```python
from build123d import *

# Parameters (mm, degrees)
SKETCH1_R           = 1.5
BOSS_EXTRUDE1_DEPTH = 5
SKETCH2_R           = 2
CUT_EXTRUDE1_DEPTH  = 5
FILLET1_R           = 7
FILLET2_R           = 7
FILLET3_R           = 3


with BuildPart() as part:
    # Sketch1 → Boss-Extrude1 (new body)
    with BuildSketch(Plane.XY):
        Polygon((33, 0), (195.6, 0), (195.6, -70), (228.6, -70), (228.6, -158.6), (195.6, -158.6), (195.6, -228.6), (33, -228.6), (33, -158.6), (0, -158.6), (0, -70), (33, -70), align=None)
        with Locations((95.3, -32)):
            Circle(SKETCH1_R, mode=Mode.SUBTRACT)
        with Locations((133.3, -32)):
            Circle(SKETCH1_R, mode=Mode.SUBTRACT)
        with Locations((39, -21.625)):
            Circle(SKETCH1_R, mode=Mode.SUBTRACT)
        with Locations((39, -38.375)):
            Circle(SKETCH1_R, mode=Mode.SUBTRACT)
        with Locations((54, -38.375)):
            Circle(SKETCH1_R, mode=Mode.SUBTRACT)
        with Locations((54, -21.625)):
            Circle(SKETCH1_R, mode=Mode.SUBTRACT)
        with Locations(Location((54, -206.975, 0), (0, 0, 180))):
            Circle(SKETCH1_R, mode=Mode.SUBTRACT)
        with Locations(Location((54, -190.225, 0), (0, 0, 180))):
            Circle(SKETCH1_R, mode=Mode.SUBTRACT)
        with Locations(Location((39, -190.225, 0), (0, 0, 180))):
            Circle(SKETCH1_R, mode=Mode.SUBTRACT)
        with Locations(Location((39, -206.975, 0), (0, 0, 180))):
            Circle(SKETCH1_R, mode=Mode.SUBTRACT)
        with Locations((174.6, -190.225)):
            Circle(SKETCH1_R, mode=Mode.SUBTRACT)
        with Locations((174.6, -206.975)):
            Circle(SKETCH1_R, mode=Mode.SUBTRACT)
        with Locations((189.6, -206.975)):
            Circle(SKETCH1_R, mode=Mode.SUBTRACT)
        with Locations((189.6, -190.225)):
            Circle(SKETCH1_R, mode=Mode.SUBTRACT)
        with Locations(Location((189.6, -38.375, 0), (0, 0, 180))):
            Circle(SKETCH1_R, mode=Mode.SUBTRACT)
        with Locations(Location((174.6, -38.375, 0), (0, 0, 180))):
            Circle(SKETCH1_R, mode=Mode.SUBTRACT)
        with Locations(Location((174.6, -21.625, 0), (0, 0, 180))):
            Circle(SKETCH1_R, mode=Mode.SUBTRACT)
        with Locations(Location((189.6, -21.625, 0), (0, 0, 180))):
            Circle(SKETCH1_R, mode=Mode.SUBTRACT)
        with BuildLine():
            Line((72.264776933, -37.198562168), (72.264776933, -22.801437832))
            ThreePointArc((72.264776933, -22.801437832), (77.438501315, -17.627713451), (82.612225696, -22.801437832))
            Line((82.612225696, -22.801437832), (82.612225696, -37.198562168))
            ThreePointArc((82.612225696, -37.198562168), (77.438501315, -42.372286549), (72.264776933, -37.198562168))
        make_face(mode=Mode.SUBTRACT)
        with BuildLine():
            Line((103.657302093, -26.446561828), (124.942697907, -26.446561828))
            ThreePointArc((124.942697907, -26.446561828), (130.496136079, -32), (124.942697907, -37.553438172))
            Line((124.942697907, -37.553438172), (103.657302093, -37.553438172))
            ThreePointArc((103.657302093, -37.553438172), (98.103863921, -32), (103.657302093, -26.446561828))
        make_face(mode=Mode.SUBTRACT)
        with BuildLine():
            Line((72.264776933, -191.401437832), (72.264776933, -205.798562168))
            ThreePointArc((72.264776933, -205.798562168), (77.438501315, -210.972286549), (82.612225696, -205.798562168))
            Line((82.612225696, -205.798562168), (82.612225696, -191.401437832))
            ThreePointArc((82.612225696, -191.401437832), (77.438501315, -186.227713451), (72.264776933, -191.401437832))
        make_face(mode=Mode.SUBTRACT)
        with BuildLine():
            Line((156.335223067, -191.401437832), (156.335223067, -205.798562168))
            ThreePointArc((156.335223067, -205.798562168), (151.161498685, -210.972286549), (145.987774304, -205.798562168))
            Line((145.987774304, -205.798562168), (145.987774304, -191.401437832))
            ThreePointArc((145.987774304, -191.401437832), (151.161498685, -186.227713451), (156.335223067, -191.401437832))
        make_face(mode=Mode.SUBTRACT)
        with BuildLine():
            Line((156.335223067, -37.198562168), (156.335223067, -22.801437832))
            ThreePointArc((156.335223067, -22.801437832), (151.161498685, -17.627713451), (145.987774304, -22.801437832))
            Line((145.987774304, -22.801437832), (145.987774304, -37.198562168))
            ThreePointArc((145.987774304, -37.198562168), (151.161498685, -42.372286549), (156.335223067, -37.198562168))
        make_face(mode=Mode.SUBTRACT)
    extrude(amount=BOSS_EXTRUDE1_DEPTH)

    # Sketch2 → Cut-Extrude1 (cut)
    with BuildSketch(Plane.XY.offset(5)):
        with Locations((54.3, -59.307305139)):
            Circle(SKETCH2_R)
        with Locations(Location((174.3, -59.307305139, 0), (0, 0, 180))):
            Circle(SKETCH2_R)
        with Locations((174.3, -169.292694861)):
            Circle(SKETCH2_R)
        with Locations(Location((54.3, -169.292694861, 0), (0, 0, 180))):
            Circle(SKETCH2_R)
    extrude(amount=-CUT_EXTRUDE1_DEPTH, mode=Mode.SUBTRACT)

    # Fillet1
    fillet1_edges = [part.edges().sort_by_distance(p)[0] for p in [
        (33, 0, 2.5),
        (195.6, 0, 2.5),
        (228.6, -70, 2.5),
        (228.6, -158.6, 2.5),
        (0, -158.6, 2.5),
        (0, -70, 2.5),
    ]]
    fillet(fillet1_edges, radius=FILLET1_R)

    # Fillet2
    fillet2_edges = [part.edges().sort_by_distance(p)[0] for p in [
        (195.6, -228.6, 2.5),
        (33, -228.6, 2.5),
    ]]
    fillet(fillet2_edges, radius=FILLET2_R)

    # Fillet3
    fillet3_edges = [part.edges().sort_by_distance(p)[0] for p in [
        (33, -70, 2.5),
        (195.6, -70, 2.5),
        (195.6, -158.6, 2.5),
        (33, -158.6, 2.5),
    ]]
    fillet(fillet3_edges, radius=FILLET3_R)


solid = part.part
```
Geometry check sheet. Reference: the model listing, model coordinates, mm. A direction names the side the tool comes from. Coordinates: 2 decimals unless noted, no trailing zeros. Order: outer loops, then holes, each group sorted by start corner. A loop starts at its lowest first (then second) coordinate and runs counter-clockwise, first axis right, second up. Notation, with made-up numbers: (59, 43.5) - (116, 43.5) arc R18 cw to (116, 53.5) - close; hole circle Ø1 at (-6.5, 33). An arc over 180 degrees is marked (long way). Answer in a Markdown table with one row per item. Add a question column.
1. Section check C-C (x = 26.5). Enter the section's corners in (y, z).
2. Access from +Z, -Z, +X, -X, +Y, -Y to the whole of each face (thin tool, end or side, straight path). Record for faces 1 (the face through (156.335, -30, 2)), 2 (the face through (33, -37, 2)), 3 (the face through (19, -158.6, 2)), 4 (the face through (195.6, -37, 2)), 5 (the face through (195.6, -191, 2)).
3. Section check B-B (y = -183.5). Enter the section's corners in (x, z).
4. Gauge pin test, flat ends, axial feed: pin 1 Ø2.5 at (x, z) = (24, 2) entering from +Y; pin 2 Ø2.5 at (y, z) = (-200, 1.5) entering from +X; pin 3 Ø2 at (y, z) = (-75.5, 2) entering from -X. Record the tip position at first contact, or that the pin passes through.
5. Section check D-D (z = 3.8). Give the number of separate pieces and of enclosed holes in the cut face, plus the area to 3 significant figures.
6. Section check A-A (x = 153). Enter the section's corners in (y, z), plus the area to 3 significant figures.
7. Draft check along Y on faces 6 (the face through (113, 0, 2)), 7 (the face through (151.28, -17.63, 2.46)), 8 (the face through (35, -226.5, 2.5)). Enter one of: +Y half, -Y half, draft (parallel to the pull), parting line (faces both ways), or undercut.
8. Material ranges on L1, parallel to X at y = -59, z = 3.2; L2, parallel to Y at x = 150.5, z = 3.15; L3, parallel to X at y = -200, z = 4.4, recorded low to high. Write a range as [from, to].
Data:
| question | item | result |
|---|---|---|
| 1 | outline | (-158.6, 0) - (-70, 0) - (-70, 5) - (-158.6, 5) - close |
| 2 | face 1 | +Z, -Z |
| 2 | face 2 | +Z, -Z, -X, +Y |
| 2 | face 3 | +Z, -Z, -X, -Y |
| 2 | face 4 | +Z, -Z, +X, +Y |
| 2 | face 5 | +Z, -Z, +X, -Y |
| 3 | outline | (33, 0) - (195.6, 0) - (195.6, 5) - (33, 5) - close |
| 4 | pin 1 | stops at y = -70 |
| 4 | pin 2 | stops at x = 195.6 |
| 4 | pin 3 | stops at x = 0.02 |
| 5 | separate pieces | 1 |
| 5 | enclosed holes | 27 |
| 5 | area | 41,500 mm² |
| 6 | outline | (-228.6, 0) - (-210.63, 0) - (-210.63, 5) - (-228.6, 5) - close; (-186.57, 0) - (-42.03, 0) - (-42.03, 5) - (-186.57, 5) - close; (-17.97, 0) - (0, 0) - (0, 5) - (-17.97, 5) - close |
| 6 | area | 902 mm² |
| 7 | face 6 | +Y half |
| 7 | face 7 | undercut |
| 7 | face 8 | -Y half |
| 8 | L1 | x = [33, 52.32], [56.28, 172.32], [176.28, 195.6] |
| 8 | L2 | y = [-228.6, -210.93], [-186.27, -42.33], [-17.67, 0] |
| 8 | L3 | x = [33, 72.26], [82.61, 145.99], [156.34, 195.6] |
